from build123d import *

# Parameters (mm, degrees)
P_IDAT_VYSUNUT_M1_DEPTH  = 3
SKICA2_W                 = 3
SKICA2_H                 = 5
ODEBRAT_VYSUNUT_M1_DEPTH = 100.328998787
SKICA3_W                 = 25
SKICA3_H                 = 3
SKICA3_W_2               = 3
SKICA3_H_2               = 5
P_IDAT_VYSUNUT_M2_DEPTH  = 3
SKICA4_R                 = 2
ODEBRAT_VYSUNUT_M3_DEPTH = 103.011028816


with BuildPart() as part:
    # Skica1 → Přidat vysunutím1 (new body)
    with BuildSketch(Plane(origin=(0, 0, 0), x_dir=(1, 0, 0), z_dir=(0, 1, 0))):
        Polygon((-88.5, 0), (88.5, 0), (88.5, -45), (45, -45), (15, -25), (-88.5, -25), align=None)
    extrude(amount=P_IDAT_VYSUNUT_M1_DEPTH)

    # Skica2 → Odebrat vysunutím1 (cut, through all)
    with BuildSketch(Plane(origin=(0, 0, 0), x_dir=(1, 0, 0), z_dir=(0, 1, 0))):
        with Locations((0, -7.5)):
            Rectangle(SKICA2_W, SKICA2_H)
        with Locations((0, -17.5)):
            Rectangle(SKICA2_W, SKICA2_H)
        with Locations((-66.5, -7.5)):
            Rectangle(SKICA2_W, SKICA2_H)
        with Locations((-66.5, -17.5)):
            Rectangle(SKICA2_W, SKICA2_H)
        with Locations((66.5, -7.5)):
            Rectangle(SKICA2_W, SKICA2_H)
        with Locations((66.5, -17.5)):
            Rectangle(SKICA2_W, SKICA2_H)
        with Locations((66.5, -27.5)):
            Rectangle(SKICA2_W, SKICA2_H)
        with Locations((66.5, -37.5)):
            Rectangle(SKICA2_W, SKICA2_H)
    extrude(amount=ODEBRAT_VYSUNUT_M1_DEPTH, mode=Mode.SUBTRACT)

    # Skica3 → Přidat vysunutím2 (add)
    with BuildSketch(Plane(origin=(0, 0, 0), x_dir=(1, 0, 0), z_dir=(0, 1, 0))):
        with Locations((-50, 1.5)):
            Rectangle(SKICA3_W, SKICA3_H)
        with Locations((0, 1.5)):
            Rectangle(SKICA3_W, SKICA3_H)
        with Locations((50, 1.5)):
            Rectangle(SKICA3_W, SKICA3_H)
        with Locations((90, -7.5)):
            Rectangle(SKICA3_W_2, SKICA3_H_2)
        with Locations((-90, -7.5)):
            Rectangle(SKICA3_W_2, SKICA3_H_2)
    extrude(amount=P_IDAT_VYSUNUT_M2_DEPTH)

    # Skica4 → Odebrat vysunutím3 (cut, through all)
    with BuildSketch(Plane(origin=(0, 0, 0), x_dir=(1, 0, 0), z_dir=(0, 1, 0))):
        with Locations(Location((-78.65, -12.27, 0), (0, 0, 90))):
            Circle(SKICA4_R)
        with Locations(Location((78.83, -35.13, 0), (0, 0, 90))):
            Circle(SKICA4_R)
    extrude(amount=ODEBRAT_VYSUNUT_M3_DEPTH, mode=Mode.SUBTRACT)


solid = part.part
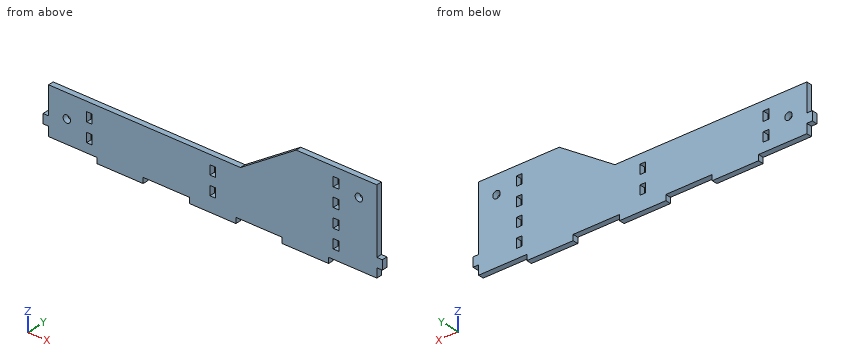
Input: part model. Units: mm. Frame: model coordinates. Give positions to 0.01 mm unless a question says otherwise; leave off trailing zeros. Loops run counter-clockwise (first coordinate to the right, second up) from the corner with the lowest first, then second, coordinate; pieces in that order, holes last. Notation, with made-up numbers: (72.5, 52) - (103.5, 52) arc R12 cw to (103.5, 63) - close; hole circle Ø5 at (64.5, 68.25). An arc over 180 degrees is marked (long way). Use CSV: the item, a comma, the result in double quotes. Start each with the question number.
Item 1: Section D-D on x = -8. Return loops of the section in (y, z).
Item 2: Section B-B on x = 78.83. Return loops of the section in (y, z), then the cut area to 3 significant figures.
Item 3: Section A-A on z = 27. Return loops of the section in (x, y), then the cut area to 4 significant figures.
Item 4: Line query: line 1 (X direction, y = 1.7, z = 6.5); line 2 (X direction, y = 1.75, z = 17); line 3 (Z direction, x = -66, y = 1.95). Output: solid intervals per line, ascending.
Item 5: Section C-C on y = 2.15. State how many separate pieces and enclosed holes the cut face has, then the cut area to 3 significant figures.
Item 6: Contact query for flat-ended pins moving along their axis: P1, Ø1.5, axis at x = -34.5, y = 1, coming from the +Z side; P2, Ø1.5, axis at x = -89.5, y = 1.5, coming from the +Z side; P3, Ø0.9, axis at y = 2, z = 16.5, coming from the +X side. Output: stop coordinate, or through.
Ans:
1,outline,"(0, -3) - (3, -3) - (3, 25) - (0, 25) - close"
2,outline,"(0, 0) - (3, 0) - (3, 33.13) - (0, 33.13) - close; (0, 37.13) - (3, 37.13) - (3, 45) - (0, 45) - close"
2,area,"123 mm2"
3,outline,"(18, 0) - (65, 0) - (65, 3) - (18, 3) - close; (68, 0) - (88.5, 0) - (88.5, 3) - (68, 3) - close"
3,area,"202.5 mm2"
4,line 1,"x = -91.5 to -68, -65 to -1.5, 1.5 to 65, 68 to 91.5"
4,line 2,"x = -88.5 to -68, -65 to -1.5, 1.5 to 65, 68 to 88.5"
4,line 3,"z = 0 to 5, 10 to 15, 20 to 25"
5,separate pieces,"1"
5,enclosed holes,"10"
5,area,"5,700 mm2"
6,P1,"stops at z = 25"
6,P2,"stops at z = 10"
6,P3,"stops at x = 88.5"
